Verification items for this drawing (mm, ordinates from the low corner). A direction names the side the tool comes from. Round coordinates to 2 decimals unless told otherwise and drop trailing zeros. Order: outer loops, then holes, each group sorted by start corner. A loop starts at its lowest first (then second) coordinate and runs counter-clockwise, first axis right, second up. Notation, with made-up numbers: (-5.5, -25) -> (2.5, -25) arc R21 cw to (2.5, -14) -> close; hole circle Ø5 at (-25.75, 82.5). An arc over 180 degrees is marked (long way). Return JSON: item names as keys, results as strings. Group by question number.
Item 1: Access from +Z, -Z, +X, -X, +Y, -Y to the whole of each face (thin tool, end or side, straight path). Record for the marked faces 3 and 4.
Item 2: Scan lines: probe 1 along Y at (x, z) = (8, 2.1); probe 2 along X at (y, z) = (6.75, 2.5); probe 3 along Z at (x, y) = (74, 24.5) (1 decimal). Record each from-to range of solid material in increasing order. Write a range as from..to.
Item 3: Depth check by flat-ended pin: pin 1 Ø3.5 at (x, y) = (8, 8) entering from +Z; pin 2 Ø11.5 at (x, y) = (47.5, 17.5) entering from +Z (3 decimals); pin 3 Ø1.6 at (y, z) = (24, 1) entering from -X; pin 4 Ø0.9 at (y, z) = (27.5, 1.5) entering from +X. Enter the tip coordinate at first touch or a pass-through.
Item 4: Sectioned sample at D-D on y = 20.5. Record the cut outline in (x, z) (1 decimal).
Item 5: Sectioned sample at B-B on y = 8. Record the cut outline in (x, z) (1 decimal).
Item 6: Sectioned sample at C-C on x = 80. Record the cut outline in (y, z) (1 decimal).
Item 7: Draft check along X on the marked faces 1 and 2. Enter one of: pulls with the +X half, pulls with the -X half, needs draft (parallel to the pull), parting line crosses it, or undercut.
Item 8: Sectioned sample at A-A on z = 1.1. Record the cut outline in (x, y), plus the area to 3 significant figures.
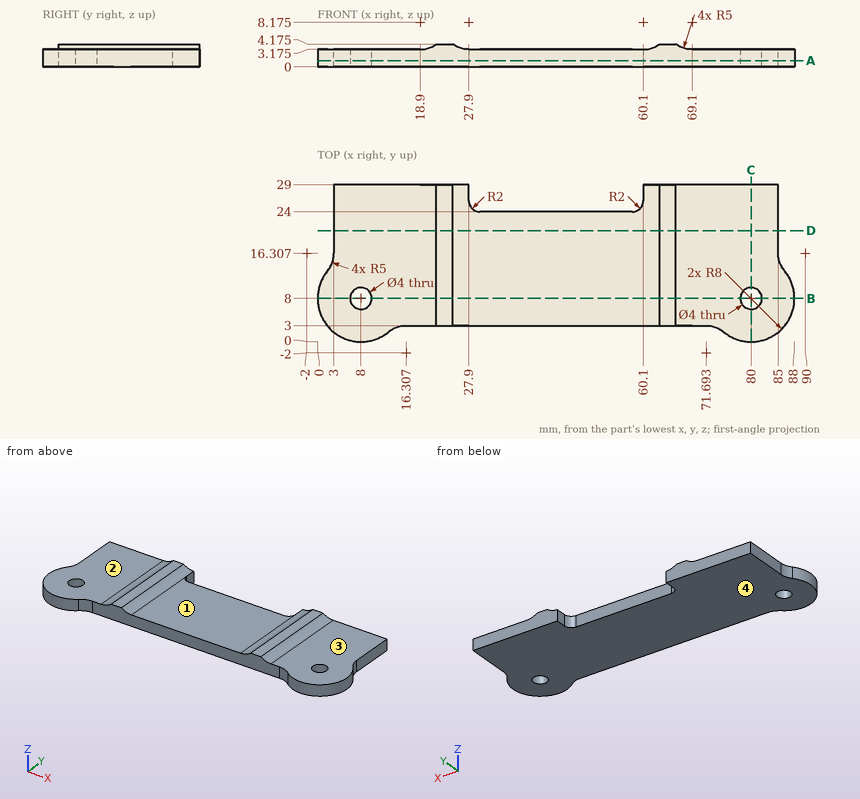
Recorded:
{
 "1": {"face 3": "+Z, +X, +Y, -Y", "face 4": "-Z, +X, -X, +Y, -Y"},
 "2": {"probe 1": "0..6, 10..29", "probe 2": "0.1..6.44, 9.56..78.44, 81.56..87.9", "probe 3": "0..3.2"},
 "3": {"pin 1": "through", "pin 2": "z = 3.175", "pin 3": "x = 3", "pin 4": "x = 85"},
 "4": {"outline": "(3, 0) -> (85, 0) -> (85, 3.2) -> (69.1, 3.2) arc R5 cw to (66.1, 4.2) -> (63.1, 4.2) arc R5 cw to (60.1, 3.2) -> (27.9, 3.2) arc R5 cw to (24.9, 4.2) -> (21.9, 4.2) arc R5 cw to (18.9, 3.2) -> (3, 3.2) -> close"},
 "5": {"outline": "(0, 0) -> (6, 0) -> (6, 3.2) -> (0, 3.2) -> close; (10, 0) -> (78, 0) -> (78, 3.2) -> (69.1, 3.2) arc R5 cw to (66.1, 4.2) -> (63.1, 4.2) arc R5 cw to (60.1, 3.2) -> (27.9, 3.2) arc R5 cw to (24.9, 4.2) -> (21.9, 4.2) arc R5 cw to (18.9, 3.2) -> (10, 3.2) -> close; (82, 0) -> (88, 0) -> (88, 3.2) -> (82, 3.2) -> close"},
 "6": {"outline": "(0, 0) -> (6, 0) -> (6, 3.2) -> (0, 3.2) -> close; (10, 0) -> (29, 0) -> (29, 3.2) -> (10, 3.2) -> close"},
 "7": {"face 1": "undercut", "face 2": "needs draft"},
 "8": {"outline": "(1.85, 13.11) arc R8 ccw to (13.11, 1.85) arc R5 cw to (16.31, 3) -> (71.69, 3) arc R5 cw to (74.89, 1.85) arc R8 ccw to (86.15, 13.11) arc R5 cw to (85, 16.31) -> (85, 29) -> (60.1, 29) -> (60.1, 26) arc R2 cw to (58.1, 24) -> (29.9, 24) arc R2 cw to (27.9, 26) -> (27.9, 29) -> (3, 29) -> (3, 16.31) arc R5 cw to start; hole circle Ø4 at (8, 8); hole circle Ø4 at (80, 8)", "area": "2,050 mm²"}
}
